The drawing under review shows one solid part. Ordinate dimensions are in mm from its lowest x, y, z. A direction names the side the tool comes from. Give positions to 0.01 mm unless a question says otherwise; leave off trailing zeros. Order: outer loops, then holes, each group sorted by start corner. A loop starts at its lowest first (then second) coordinate and runs counter-clockwise, first axis right, second up. Notation, with made-up numbers: (20.25, 50.5) - (57.25, 50.5) arc R25 ccw to (57.25, 71.5) - close; hole circle Ø3 at (35.25, 14.25). An arc over 180 degrees is marked (long way). Use CSV: the item, a comma, the result in double quotes. Start each with the question number.
1. Take a section at A-A, the plane y = 8. State the section outline as (x, z) points, then the cut area to 3 significant figures.
2. Take a section at D-D, the plane z = 1.25. State the section outline as (x, y) points, then the cut area to 3 significant figures.
3. To check wall thickness, follow line 1 (Y direction, x = 8, z = 4); line 2 (Z direction, x = 3, y = 12); line 3 (Y direction, x = 7.25, z = 1.25). State the ranges of each line that lie inside material, in increasing order. Write a range as [from, to].
4. Draft analysis for pull direction Y (two halves, no side actions). For the marked faces 1, 2 and 3, state which applies: released by +Y, released by -Y, zero draft, split by the parting line, or undercut.
5. Take a section at C-C, the plane z = 3.25. State the section outline as (x, y) points.
6. Machinability: for the marked faces 4 and 5, which of the approach directions +Z, -Z, +X, -X, +Y, -Y give a long, thin tool a straight path to every point of the face, cutting with its end or side? Answer none if there is none.
7. For pin 1 (1 mm diameter, centred on x = 11.5, y = 5.5, fed in from -Z); pin 2 (4 mm diameter, centred on x = 13.5, z = 4.5, fed in from +Y); pin 3 (2 mm diameter, centred on y = 3, z = 5, fed in from +X); pin 4 (3 mm diameter, centred on x = 3, z = 5.5, fed in from -Y), all flat-tipped, find the tip position at first contact; note any pin that passes through.
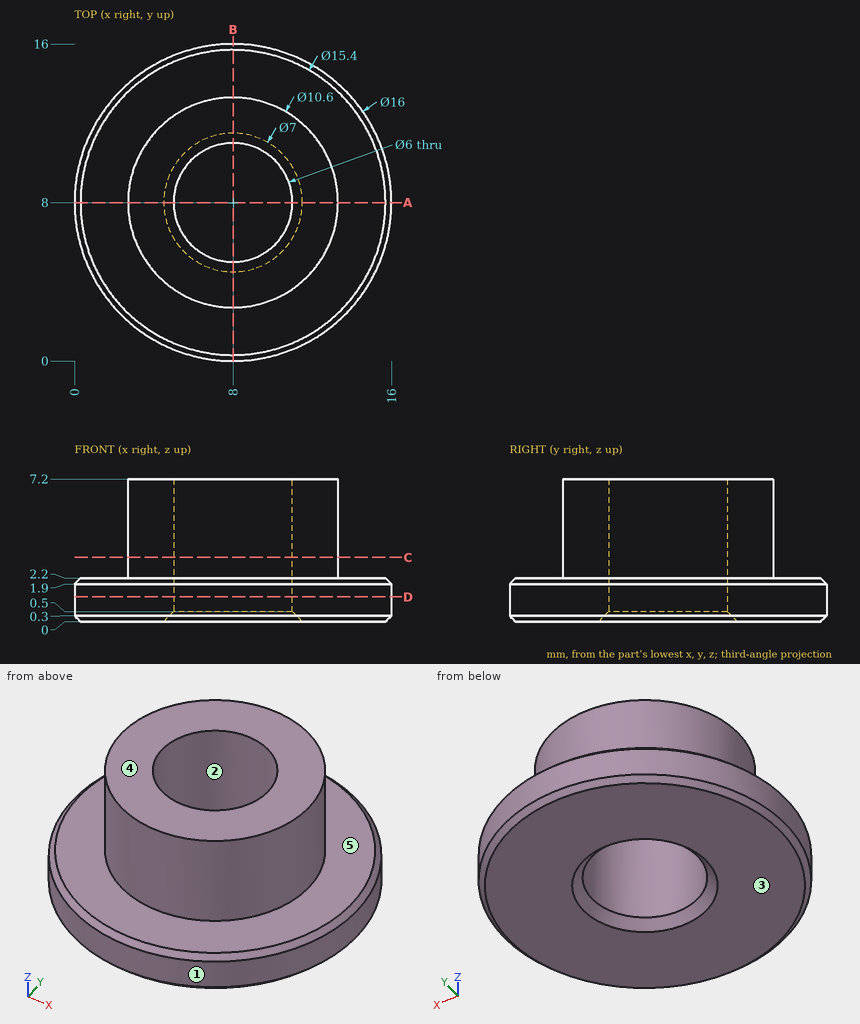
Determined:
1,outline,"(0, 0.3) - (0.3, 0) - (4.5, 0) - (5, 0.5) - (5, 7.2) - (2.7, 7.2) - (2.7, 2.2) - (0.3, 2.2) - (0, 1.9) - close; (11, 0.5) - (11.5, 0) - (15.7, 0) - (16, 0.3) - (16, 1.9) - (15.7, 2.2) - (13.3, 2.2) - (13.3, 7.2) - (11, 7.2) - close"
1,area,"44.6 mm²"
2,outline,"circle Ø16 at (8, 8); hole circle Ø6 at (8, 8)"
2,area,"173 mm²"
3,line 1,"y = [2.7, 5], [11, 13.3]"
3,line 2,"z = [0, 2.2]"
3,line 3,"y = [0.04, 5.1], [10.9, 15.96]"
4,face 1,"split by the parting line"
4,face 2,"undercut"
4,face 3,"zero draft"
5,outline,"circle Ø10.6 at (8, 8); hole circle Ø6 at (8, 8)"
6,face 4,"+Z, +X, -X, +Y, -Y"
6,face 5,"+Z"
7,pin 1,"stops at z = 0"
7,pin 2,"stops at y = 11.98"
7,pin 3,"stops at x = 11.48"
7,pin 4,"stops at y = 4.02"
